For this review, take the finished solid that the model builds, in its own axes (mm). Face numbers are marked on the shaded views. A direction names the side the tool comes from. Round coordinates to 2 decimals unless told otherwise and drop trailing zeros. Order: outer loops, then holes, each group sorted by start corner. A loop starts at its lowest first (then second) coordinate and runs counter-clockwise, first axis right, second up. Notation, with made-up numbers: M 58,33.5 L 64,33.5 A4 cw 64,37.5 Z; hole C 36,20 d9. An arc over 180 degrees is marked long. Answer as a JSON object with one key per item and string values.
from build123d import *

# Parameters (mm, degrees)
F0_W     = 93
F0_H     = 63
F1_DEPTH = 15
F2_T     = -2.5
F3_W     = 90
F3_H     = 60
F4_DEPTH = 3.5
F6_DEPTH = 2
F7_SIZE  = 0.2
F9_DEPTH = 93.001
F10_SIZE = 0.4


with BuildPart() as f1:
    # F0 (on Top) → F1 (new body)
    with BuildSketch(Plane.XY):
        Rectangle(F0_W, F0_H)
    extrude(amount=-F1_DEPTH)

    # F2
    f2_openings = [f1.faces().sort_by_distance(p)[0] for p in [
        (0, 0, 0),
    ]]
    offset(amount=F2_T, openings=f2_openings)

    # F3 (on Top) → F4 (cut)
    with BuildSketch(Plane.XY):
        Rectangle(F3_W, F3_H)
    extrude(amount=-F4_DEPTH, mode=Mode.SUBTRACT)

    # F5 (on face) → F6 (join)
    with BuildSketch(Plane.XY.offset(-12.5)):
        Polygon((-42, 19), (-42, 27), (-34, 27), (-36.1213203436, 24.8786796564), (-35.4142135624, 24.1715728753), (-31.5857864376, 28), (-43, 28), (-43, 16.5857864376), (-39.1715728753, 20.4142135624), (-39.8786796564, 21.1213203436), align=None)
        Polygon((34, 27), (42, 27), (42, 19), (39.8786796564, 21.1213203436), (39.1715728753, 20.4142135624), (43, 16.5857864376), (43, 28), (31.5857864376, 28), (35.4142135624, 24.1715728753), (36.1213203436, 24.8786796564), align=None)
        Polygon((-43, -16.5857864376), (-43, -28), (-31.5857864376, -28), (-35.4142135624, -24.1715728753), (-36.1213203436, -24.8786796564), (-34, -27), (-42, -27), (-42, -19), (-39.8786796564, -21.1213203436), (-39.1715728753, -20.4142135624), align=None)
        Polygon((31.5857864376, -28), (43, -28), (43, -16.5857864376), (39.1715728753, -20.4142135624), (39.8786796564, -21.1213203436), (42, -19), (42, -27), (34, -27), (36.1213203436, -24.8786796564), (35.4142135624, -24.1715728753), align=None)
    extrude(amount=F6_DEPTH)

    # F7
    f7_edges = [f1.edges().sort_by_distance(p)[0] for p in [
        (-39.525126, 20.767767, -10.5),
        (-40.93934, 20.06066, -10.5),
        (-42, 23, -10.5),
        (-38, 27, -10.5),
        (-35.06066, 25.93934, -10.5),
        (-35.767767, 24.525126, -10.5),
        (-33.5, 26.085786, -10.5),
        (-37.292893, 28, -10.5),
        (-43, 22.292893, -10.5),
        (-41.085786, 18.5, -10.5),
        (35.767767, 24.525126, -10.5),
        (35.06066, 25.93934, -10.5),
        (38, 27, -10.5),
        (42, 23, -10.5),
        (40.93934, 20.06066, -10.5),
        (39.525126, 20.767767, -10.5),
        (41.085786, 18.5, -10.5),
        (43, 22.292893, -10.5),
        (37.292893, 28, -10.5),
        (33.5, 26.085786, -10.5),
        (33.5, -26.085786, -10.5),
        (37.292893, -28, -10.5),
        (43, -22.292893, -10.5),
        (41.085786, -18.5, -10.5),
        (39.525126, -20.767767, -10.5),
        (40.93934, -20.06066, -10.5),
        (42, -23, -10.5),
        (38, -27, -10.5),
        (35.06066, -25.93934, -10.5),
        (35.767767, -24.525126, -10.5),
        (-41.085786, -18.5, -10.5),
        (-43, -22.292893, -10.5),
        (-37.292893, -28, -10.5),
        (-33.5, -26.085786, -10.5),
        (-35.767767, -24.525126, -10.5),
        (-35.06066, -25.93934, -10.5),
        (-38, -27, -10.5),
        (-42, -23, -10.5),
        (-40.93934, -20.06066, -10.5),
        (-39.525126, -20.767767, -10.5),
    ]]
    chamfer(f7_edges, length=F7_SIZE)

    # F8 (on face) → F9 (cut, through all)
    with BuildSketch(Plane.YZ.offset(46.5)):
        with BuildLine():
            Line((-8, 0), (-8, -3.5))
            ThreePointArc((-8, -3.5), (0, -9.0440037453), (8, -3.5))
            Line((8, -3.5), (8, 0))
            Line((8, 0), (0, 0))
            Line((0, 0), (-8, 0))
        make_face()
    extrude(amount=-F9_DEPTH, mode=Mode.SUBTRACT)

    # F10
    f10_edges = [f1.edges().sort_by_distance(p)[0] for p in [
        (46.5, 0, -9.044004),
        (46.5, 8, -1.75),
        (46.5, -8, -1.75),
        (-46.5, 8, -1.75),
        (-46.5, 0, -9.044004),
        (-46.5, -8, -1.75),
    ]]
    chamfer(f10_edges, length=F10_SIZE)


solid = f1.part
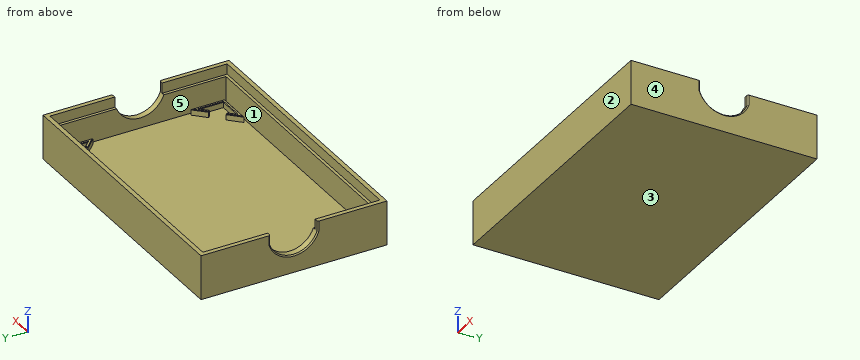
1) Add section B-B on x = -37.5. State the section outline as (y, z) points.
Geometry check:
{"outline": "M -31.5,-15 L 31.5,-15 L 31.5,0 L 30,0 L 30,-3.5 L 29,-3.5 L 29,-12.5 L 28,-12.5 L 28,-10.7 L 27.8,-10.5 L 27.2,-10.5 L 27,-10.7 L 27,-12.5 L -27,-12.5 L -27,-10.7 L -27.2,-10.5 L -27.8,-10.5 L -28,-10.7 L -28,-12.5 L -29,-12.5 L -29,-3.5 L -30,-3.5 L -30,0 L -31.5,0 Z"}
2) Add section A-A on z = -1.5. State the section outline as (x, y) points.
Geometry check:
{"outline": "M -46.5,-31.5 L 46.5,-31.5 L 46.5,-8.4 L 46.1,-8 L 45,-8 L 45,-30 L -45,-30 L -45,-8 L -46.1,-8 L -46.5,-8.4 Z; M -46.5,8.4 L -46.1,8 L -45,8 L -45,30 L 45,30 L 45,8 L 46.1,8 L 46.5,8.4 L 46.5,31.5 L -46.5,31.5 Z"}
3) For L1, parallel to X at y = -17.5, z = -7; L2, parallel to Y at x = 6, z = -6.5; L3, parallel to Y at x = -29, z = -1.25, list the stretches that pass through material, from the lowest coordinate up.
Geometry check:
{"L1": "x = -46.5 to -44, 44 to 46.5", "L2": "y = -31.5 to -29, 29 to 31.5", "L3": "y = -31.5 to -30, 30 to 31.5"}
4) Insertion check: P1, Ø3, axis at x = 38.5, y = -23, coming from the +Z side. The pin has a flat end and moves straight along its axis. Give the tip position at first contact, or say it passes through.
Geometry check:
{"P1": "stops at z = -12.5"}
5) Machinability: for the marked faces 4 and 5, which of the approach directions +Z, -Z, +X, -X, +Y, -Y give a long, thin tool a straight path to every point of the face, cutting with its end or side? Answer none if there is none.
Geometry check:
{"face 4": "+Z, -Z, +X, +Y, -Y", "face 5": "+Z"}
6) Add section C-C on y = 22.5. State the section outline as (x, z) points, and give its area (3 significant figures).
Geometry check:
{"outline": "M -46.5,-15 L 46.5,-15 L 46.5,0 L 45,0 L 45,-3.5 L 44,-3.5 L 44,-12.5 L 43,-12.5 L 43,-10.7 L 42.8,-10.5 L 42.2,-10.5 L 42,-10.7 L 42,-12.5 L -42,-12.5 L -42,-10.7 L -42.2,-10.5 L -42.8,-10.5 L -43,-10.7 L -43,-12.5 L -44,-12.5 L -44,-3.5 L -45,-3.5 L -45,0 L -46.5,0 Z", "area": "292 mm²"}
7) Mouldability with a two-part tool opening along Y and no side actions: class the marked faces 1, 2 and 3 as +Y half, -Y half, draft (parallel to the pull), parting line (faces both ways), or undercut.
Geometry check:
{"face 1": "undercut", "face 2": "-Y half", "face 3": "draft"}
8) Add section D-D on x = 14. State the section outline as (y, z) points.
Geometry check:
{"outline": "M -31.5,-15 L 31.5,-15 L 31.5,0 L 30,0 L 30,-3.5 L 29,-3.5 L 29,-12.5 L -29,-12.5 L -29,-3.5 L -30,-3.5 L -30,0 L -31.5,0 Z"}
